For this review, take the finished solid that the model builds, in its own axes (mm). A direction names the side the tool comes from. Give positions to 0.01 mm unless a question says otherwise; leave off trailing zeros. Write each loop counter-clockwise with the first axis right and the second up, starting at its lowest first coordinate (ties: lowest second). Pieces come first, ordered by that corner, then holes. Notation, with made-up numbers: (60.25, -30.75) -> (81.25, -30.75) arc R12 cw to (81.25, -22.75) -> close; hole circle Ø11 at (34.25, 33). An arc over 180 degrees is marked (long way). Return JSON: item names as keys, results as strings.
from build123d import *

# Parameters (mm, degrees)
PAD_DEPTH             = 0.8
POLARPATTERN_COUNT    = 3
SKETCH002_R           = 1.75
POCKET_DEPTH          = 163.720738
POLARPATTERN001_COUNT = 3


with BuildPart() as part:
    # Sketch → Revolution (revolve)
    with BuildSketch(Plane.XZ):
        Polygon((-7, 4), (7, 4), (7, 6.9), (1.5, 6.9), (1.5, 20.7), (7, 20.7), (7, 25), (6, 25), (6, 26), (-6, 26), (-6, 25), (-7, 25), (-7, 20.7), (-1.5, 20.7), (-1.5, 13), (-3.5, 13), (-3.5, 10.5), (-1.5, 10.5), (-1.5, 6.9), (-7, 6.9), align=None)
    revolve(axis=Axis((0, 0, 0), (1, 0, 0)))

    # Sketch001 (on Face4 of Revolution) → Pad (new body)
    with BuildSketch(Plane(origin=(1.5, 0, 0), x_dir=(0, 0, 1), z_dir=(1, 0, 0))):
        with BuildLine():
            Line((2, 20.603155), (2, 6.603787))
            ThreePointArc((2, 6.603787), (0, 6.9), (-2, 6.603787))
            Line((-2, 6.603787), (-2, 20.603155))
            ThreePointArc((2, 20.603155), (0, 20.7), (-2, 20.603155))
        make_face()
    pad = extrude(amount=PAD_DEPTH)

    # PolarPattern: Pad ×3 about axis
    polarpattern_axis = Axis((1.5, 0, 0), (1, 0, 0))
    for i in range(1, POLARPATTERN_COUNT):
        add(pad.rotate(polarpattern_axis, i * 360 / POLARPATTERN_COUNT))

    # Sketch002 (on Face22 of PolarPattern) → Pocket (cut, through all)
    with BuildSketch(Plane(origin=(7, 0, 0), x_dir=(0, 0, 1), z_dir=(1, 0, 0))):
        with Locations((0, 12.3)):
            Circle(SKETCH002_R)
    pocket = extrude(amount=-POCKET_DEPTH, mode=Mode.SUBTRACT)

    # PolarPattern001: Pocket ×3 about axis
    polarpattern001_axis = Axis((7, 0, 0), (1, 0, 0))
    for i in range(1, POLARPATTERN001_COUNT):
        add(pocket.rotate(polarpattern001_axis, i * 360 / POLARPATTERN001_COUNT), mode=Mode.SUBTRACT)


solid = part.part
1. Add section C-C, the plane z = 0. Count the separate pieces of the cut face and the enclosed holes in it, plus the area to 3 significant figures.
Results found:
{"separate pieces": "3", "enclosed holes": "0", "area": "311 mm²"}
2. To check wall thickness, follow probe 1 along Z at (x, y) = (-2.2, 0); probe 2 along Y at (x, z) = (1.25, 0); probe 3 along Z at (x, y) = (5, 0). State the ranges of each line that lie inside material, in increasing order.
Results found:
{"probe 1": "z = -26 to -20.7, -13 to -10.5, -6.9 to -4, 4 to 6.9, 10.5 to 13, 20.7 to 26", "probe 2": "y = -26 to -14.05, -10.55 to -4, 4 to 26", "probe 3": "z = -26 to -20.7, -6.9 to -4, 4 to 6.9, 20.7 to 26"}
3. Add section A-A, the plane x = 3.75. State the section outline as (y, z) points, plus the area to 3 significant figures.
Results found:
{"outline": "circle Ø52 at (0, 0); circle Ø13.8 at (0, 0); hole circle Ø41.4 at (0, 0); hole circle Ø8 at (0, 0)", "area": "877 mm²"}
4. The part is to be moulded in two halves that separate along Y. For faces 1 (the cylindrical face through (-0.084, 15.821, -20.633)), 2 (the cylindrical face through (-0.56, -10.75, 0.81)), 3 (the flat face through (7, -19, 9)), say which applies: +Y half, -Y half, draft (parallel to the pull), parting line (faces both ways), or undercut.
Results found:
{"face 1": "parting line", "face 2": "undercut", "face 3": "draft"}
5. Add section B-B, the plane y = 18. State the section outline as (x, z) points.
Results found:
{"outline": "(-7, -17.35) -> (-6, -17.35) -> (-6, -18.76) -> (6, -18.76) -> (6, -17.35) -> (7, -17.35) -> (7, -10.22) -> (1.5, -10.22) -> (1.5, 10.22) -> (7, 10.22) -> (7, 17.35) -> (6, 17.35) -> (6, 18.76) -> (-6, 18.76) -> (-6, 17.35) -> (-7, 17.35) -> (-7, 10.22) -> (-1.5, 10.22) -> (-1.5, -10.22) -> (-7, -10.22) -> close"}
6. For pin 1 (5 mm diameter, centred on x = 3, y = -19, fed in from -Z); pin 2 (3 mm diameter, centred on x = 3, z = -1.5, fed in from -Y); pin 3 (8 mm diameter, centred on x = 5, y = -6.5, fed in from +Z), all flat-tipped, find the tip position at first contact; note any pin that passes through.
Results found:
{"pin 1": "stops at z = -20.09", "pin 2": "stops at y = -26", "pin 3": "stops at z = 25.88"}
7. For faces 4 (the cylindrical face through (-0.559, 5.624, -8.983)), 5 (the flat face through (1.894, 5.021, 12.696)), 6 (the flat face through (-1.5, 7, 2)), list the 3-axis set-ups (+Z, -Z, +X, -X, +Y, -Y) from which the entire face can be reached by the end or side of a thin tool; tool diameter is ignored.
Results found:
{"face 4": "+X, -X", "face 5": "+X", "face 6": "-X"}
